```python
from build123d import *

# Parameters (mm, degrees)
SKETCH_1_W          = 7
SKETCH_1_H          = 30
EXTRUDE_1_DEPTH     = 4
EXTRUDE_2_DEPTH     = 30
SKETCH_3_R          = 1.5
CUT_EXTRUDE_2_DEPTH = 38.373237277
SKETCH_4_R          = 1.5
CUT_EXTRUDE_3_DEPTH = 38.362858307
SKETCH_5_R          = 14
CUT_EXTRUDE_4_DEPTH = 38.362858307
FILLET_1_R          = 2
FILLET_2_R          = 2
EXTRUDE_START       = -3.912590403
EXTRUDE_4_DEPTH     = 3.912590403


with BuildPart() as part:
    # 草圖1 → 填料-伸長1 (new body)
    with BuildSketch(Plane.XY):
        Rectangle(SKETCH_1_W, SKETCH_1_H)
    extrude(amount=EXTRUDE_1_DEPTH)

    # 草圖2 → 填料-伸長2 (add)
    with BuildSketch(Plane.XZ.offset(15)):
        Polygon((-3.5, 0), (-32.844428022, -6.237350725), (-33.657901308, -2.410259809), (-3.5, 4), align=None)
    extrude(amount=-EXTRUDE_2_DEPTH)

    # 草圖3 → 除料-伸長2 (cut, through all)
    with BuildSketch(Plane(origin=(0, 0, 0), x_dir=(-1, 0, 0), z_dir=(0, 0, -1))):
        with Locations((0, -12)):
            Circle(SKETCH_3_R)
        with Locations((0, 12)):
            Circle(SKETCH_3_R)
    extrude(amount=-CUT_EXTRUDE_2_DEPTH, mode=Mode.SUBTRACT)

    # 草圖4 → 除料-伸長3 (cut, through all)
    with BuildSketch(Plane(origin=(-0.151295449, 0, 0.711789125), x_dir=(-0.978147600733807, 0, -0.2079116908177533), z_dir=(0.2079116908177533, 0, -0.978147600733807))):
        with Locations((30.423516603, -12)):
            Circle(SKETCH_4_R)
        with Locations(Location((30.423516603, 12, 0), (0, 0, 180))):
            Circle(SKETCH_4_R)
        with Locations((6.423516603, 12)):
            Circle(SKETCH_4_R)
        with Locations(Location((6.423516603, -12, 0), (0, 0, 180))):
            Circle(SKETCH_4_R)
    extrude(amount=-CUT_EXTRUDE_3_DEPTH, mode=Mode.SUBTRACT)

    # 草圖5 → 除料-伸長4 (cut, through all)
    with BuildSketch(Plane(origin=(-0.151295449, 0, 0.711789125), x_dir=(-0.978147600733807, 0, -0.2079116908177533), z_dir=(0.2079116908177533, 0, -0.978147600733807))):
        with Locations((17.717091252, 0)):
            Circle(SKETCH_5_R)
    extrude(amount=-CUT_EXTRUDE_4_DEPTH, mode=Mode.SUBTRACT)

    # 圓角1
    fillet_1_edges = [part.edges().sort_by_distance(p)[0] for p in [
        (-33.251164665, -15, -4.323805267),
        (-33.251164665, 15, -4.323805267),
    ]]
    fillet(fillet_1_edges, radius=FILLET_1_R)

    # 圓角2
    fillet_2_edges = [part.edges().sort_by_distance(p)[0] for p in [
        (3.5, 15, 2),
        (3.5, -15, 2),
    ]]
    fillet(fillet_2_edges, radius=FILLET_2_R)

    # 草圖7 → 填料-伸長4 (add)
    with BuildSketch(Plane(origin=(-0.964768735, 0, 4.538880041), x_dir=(0.978147600733807, 0, 0.20791169081775324), z_dir=(-0.20791169081775324, 0, 0.978147600733807)).offset(EXTRUDE_START)):
        with BuildLine():
            Line((-3.752851208, 1), (-9.847302899, 1.43750871))
            ThreePointArc((-9.847302899, 1.43750871), (-11.244955297, 4.702282018), (-13.918040883, 7.040398873))
            Line((-13.918040883, 7.040398873), (-12.450847248, 12.971764494))
            ThreePointArc((-12.450847248, 12.971764494), (-13.39085333, 13.314791228), (-14.352960281, 13.589798483))
            Line((-14.352960281, 13.589798483), (-16.652344934, 7.928828115))
            ThreePointArc((-16.652344934, 7.928828115), (-20.189227207, 7.60845213), (-23.238937351, 5.788714508))
            Line((-23.238937351, 5.788714508), (-28.426613508, 9.016991352))
            ThreePointArc((-28.426613508, 9.016991352), (-29.043329173, 8.228993532), (-29.602184013, 7.398957363))
            Line((-29.602184013, 7.398957363), (-24.92883019, 3.462776556))
            ThreePointArc((-24.92883019, 3.462776556), (-25.717091252, 0), (-24.92883019, -3.462776556))
            Line((-24.92883019, -3.462776556), (-29.602184013, -7.398957363))
            ThreePointArc((-29.602184013, -7.398957363), (-29.043329173, -8.228993532), (-28.426613508, -9.016991352))
            Line((-28.426613508, -9.016991352), (-23.238937351, -5.788714508))
            ThreePointArc((-23.238937351, -5.788714508), (-20.189227207, -7.60845213), (-16.652344934, -7.928828115))
            Line((-16.652344934, -7.928828115), (-14.352960281, -13.589798483))
            ThreePointArc((-14.352960281, -13.589798483), (-13.39085333, -13.314791228), (-12.450847248, -12.971764494))
            Line((-12.450847248, -12.971764494), (-13.918040883, -7.040398873))
            ThreePointArc((-13.918040883, -7.040398873), (-11.244955297, -4.702282018), (-9.847302899, -1.43750871))
            Line((-9.847302899, -1.43750871), (-3.752851208, -1))
            ThreePointArc((-3.752851208, -1), (-3.717091252, 0), (-3.752851208, 1))
        make_face()
    extrude(amount=EXTRUDE_4_DEPTH)


solid = part.part
```
For this review, take the finished solid that the model builds, in its own axes (mm). A direction names the side the tool comes from. Coordinates: 2 decimals unless noted, no trailing zeros. Write each loop counter-clockwise with the first axis right and the second up, starting at its lowest first coordinate (ties: lowest second). Pieces come first, ordered by that corner, then holes.
(1) Wall thickness on probe 1 along Y at (x, z) = (0, 3.1); probe 2 along X at (y, z) = (-12.5, 0.5); probe 3 along Y at (x, z) = (-0.5, 0.5): over which ranges is each line inside the solid? List them lowest first.
(2) For pin 1 Ø1.5 at (x, y) = (-7.5, 9) entering from +Z; pin 2 Ø5 at (y, z) = (-6, -2) entering from -X; pin 3 Ø5 at (x, y) = (0, 12) entering from -Z; pin 4 Ø4 at (x, y) = (-26.5, 4) entering from -Z, all flat-tipped, find the tip position at first contact; note any pin that passes through.
(3) Tool access review of faces 4 (the face through (2.9, 14.43, 2.03)), 5 (the face through (-11.52, 4.66, 0.27)), 6 (the face through (-22.22, 13.28, -2.01)): name each direction out of +Z, -Z, +X, -X, +Y, -Y from which nothing blocks a thin tool from reaching the whole face with its end or side.
(4) Add section D-D on x = -7. Count the separate pieces of the cut face and the enclosed holes in it, then the cut area to 3 significant figures.
(5) Add section A-A on x = 0. Give the boundary of the cut face in (y, z).
(6) Add section C-C on y = -11.25. Give the boundary of the cut face in (x, z), then the cut area to 3 significant figures.
(7) Add section B-B on y = -4.5. Give the boundary of the cut face in (x, z), then the cut area to 3 significant figures.
(8) The part is to be moulded in two halves that separate along X. For faces 1 (the face through (-15.73, -10.72, -0.63)), 2 (the face through (0, 0, 4)), 3 (the face through (-32.67, 14.43, -4.17)), say which applies: +X half, -X half, draft (parallel to the pull), parting line (faces both ways), or undercut.
Answer sheet:
1. probe 1: y = -15 to -13.5, -10.5 to 10.5, 13.5 to 15
1. probe 2: x = -15.23 to -12.95, -11.77 to -8.12, -5.23 to -1.41, 1.41 to 3.5
1. probe 3: y = -15 to -13.41, -10.59 to 10.59, 13.41 to 15
2. pin 1: stops at z = 3.31
2. pin 2: stops at x = -33.66
2. pin 3: stops at z = 0
2. pin 4: stops at z = -5.06
3. face 4: +Z, -Z, +X, +Y
3. face 5: +Z
3. face 6: none
4. separate pieces: 5
4. enclosed holes: 0
4. area: 38.2 mm2
5. outline: (-15, 0) - (-13.5, 0) - (-13.5, 4) - (-15, 4) - close; (-10.5, 0) - (10.5, 0) - (10.5, 4) - (-10.5, 4) - close; (13.5, 0) - (15, 0) - (15, 4) - (13.5, 4) - close
6. outline: (-33.66, -2.41) - (-32.84, -6.24) - (-31.18, -5.88) - (-31.99, -2.06) - close; (-29.45, -1.52) - (-28.64, -5.34) - (-25.63, -4.7) - (-26.45, -0.88) - close; (-15.93, 1.36) - (-15.12, -2.47) - (-12.75, -1.97) - (-13.56, 1.86) - close; (-10.14, 2.59) - (-9.33, -1.24) - (-7.71, -0.89) - (-8.52, 2.93) - close; (-5.98, 3.47) - (-5.16, -0.35) - (-3.5, 0) - (-1.3, 0) - (-1.3, 4) - (-3.5, 4) - close; (1.3, 0) - (3.5, 0) - (3.5, 4) - (1.3, 4) - close
6. area: 60.6 mm2
7. outline: (-33.66, -2.41) - (-32.84, -6.24) - (-30.45, -5.73) - (-31.26, -1.9) - close; (-26.55, -0.9) - (-25.74, -4.73) - (-11.01, -1.6) - (-11.82, 2.23) - close; (-5.33, 3.61) - (-4.51, -0.22) - (-3.5, 0) - (3.5, 0) - (3.5, 4) - (-3.5, 4) - close
7. area: 102 mm2
8. face 1: undercut
8. face 2: draft
8. face 3: -X half
